Geometry: see drawing. Coordinates: mm, zero at the bounding-box minimum. Coordinates: 2 decimals unless noted, no trailing zeros. Loops run counter-clockwise (first coordinate to the right, second up) from the corner with the lowest first, then second, coordinate; pieces in that order, holes last. Notation, with made-up numbers: (-33, 44.5) - (1, 44.5) arc R25 cw to (1, 75.5) - close; hole circle Ø4 at (4.5, 38). An arc over 180 degrees is marked (long way). Use one line per item in the form item = value.
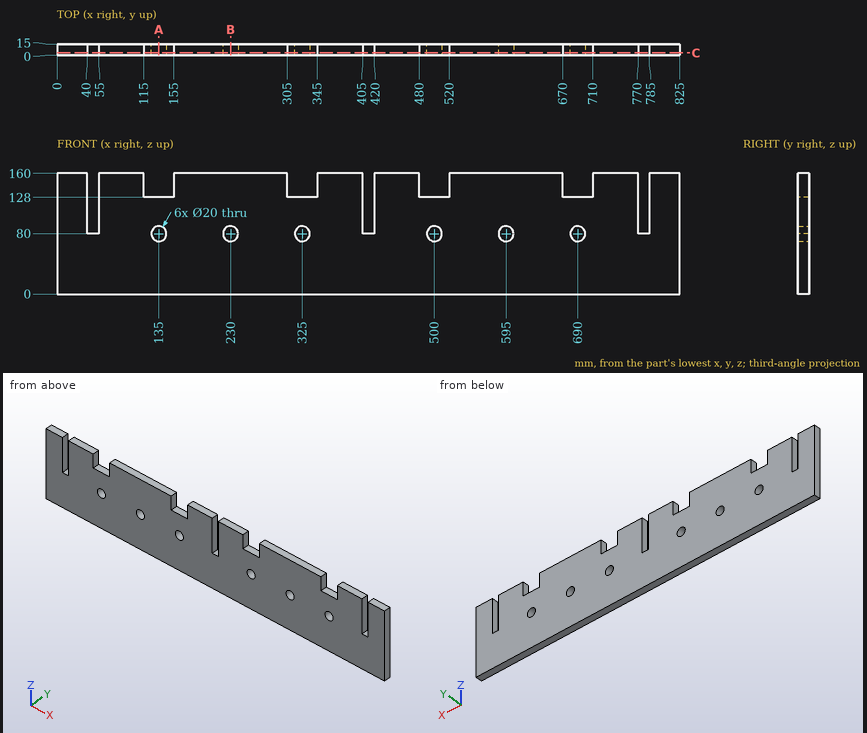
Q1. Cut plane B-B, the plane x = 230. Return loops of the section in (y, z), then the cut area to 3 significant figures.
Check values:
outline = (0, 0) - (15, 0) - (15, 70) - (0, 70) - close; (0, 90) - (15, 90) - (15, 160) - (0, 160) - close
area = 2,100 mm²
Q2. Ray query, line 1 along X through (y, z) = (9.5, 104); line 2 along Z through (x, y) = (595, 6.5); line 3 along Z through (x, y) = (325, 9.5). Return the intervals inside material, ascending. Write a range as [from, to].
Check values:
line_1 = [0, 40], [55, 405], [420, 770], [785, 825]
line_2 = [0, 70], [90, 160]
line_3 = [0, 70], [90, 128]
Q3. Cut plane C-C, the plane y = 3.25. Give the number of separate pieces and of enclosed holes in the cut face, then the cut area to 3 significant figures.
Check values:
separate_pieces = 1
enclosed_holes = 6
area = 121,000 mm²
Q4. First-contact query: P1, Ø7.5, axis at x = 780, y = 8.5, coming from the +Z side; P2, Ø4.5, axis at x = 690.5, y = 9, coming from the +Z side; P3, Ø12, axis at x = 325, z = 80, coming from the -Y side. Flat tips, straight axial feed; report the tip coordinate or a pass-through.
Check values:
P1 = 80
P2 = 128
P3 = through
Q5. Cut plane A-A, the plane x = 135. Return loops of the section in (y, z).
Check values:
outline = (0, 0) - (15, 0) - (15, 70) - (0, 70) - close; (0, 90) - (15, 90) - (15, 128) - (0, 128) - close
